CAD build for the part. Positions are in the model's coordinates, mm. A direction names the side the tool comes from. Round coordinates to 2 decimals unless told otherwise and drop trailing zeros. Order: outer loops, then holes, each group sorted by start corner. A loop starts at its lowest first (then second) coordinate and runs counter-clockwise, first axis right, second up. Notation, with made-up numbers: M 48,-30.75 L 93,-30.75 A21 cw 93,-3.75 Z; hole C -21,60 d1. An arc over 180 degrees is marked long. Put each result on its own line as item: value.
Autodesk Inventor part; units mm, degrees
ref_plane "YZ Plane" through (0, 0, 0) normal (1, 0, 0) x (0, 1, 0)
ref_plane "XZ Plane" through (0, 0, 0) normal (0, 1, 0) x (-1, 0, 0)
ref_plane "XY Plane" through (0, 0, 0) normal (0, 0, 1) x (1, 0, 0)
sketch "Sketch1" plane through (0, 0, 0) normal (0, 0, 1) x (1, 0, 0)
  circle A0 centre (-3.2581, -3.2482) radius 0.75
  circle A1 centre (11.7419, -13.2482) radius 0.75
  arc A2 (11.7419, -16.7482) -> (11.7419, -9.7482) centre (11.7419, -13.2482) ccw
  arc A3 (0.2419, -3.2482) -> (-6.7581, -3.2482) centre (-3.2581, -3.2482) ccw
  circle A4 centre (11.7419, -13.2482) radius 0.75
  circle A5 centre (-3.2581, -3.2482) radius 0.75
  line L0 (0.2419, -3.2482) -> (0.2419, -8.2482)
  line L1 (-6.7581, -3.2482) -> (-6.7581, -10.2482)
  line L2 (11.7419, -9.7482) -> (2.2419, -9.7482)
  line L3 (2.2419, -9.7482) -> (0.2419, -8.2482)
  line L4 (11.7419, -16.7482) -> (0.2419, -16.7482)
  line L5 (-6.7581, -10.2482) -> (0.2419, -16.7482)
  point P0 (0, 0)
  point P1 (-5.7424, -0.7828)
  point P2 (9.5175, -10.546)
  dimension "d0" = 7
  dimension "d1" = 7
  dimension "d4" = 5
  dimension "d5" = 7
  dimension "d6" = 9.5
  dimension "d7" = 11.5
  dimension "d8" = 15
extrude "Extrusion1" add sketch "Sketch1" against normal blind 4
properties part number "linkage"
Item 1: Mould opens along Y. For faces 1 (the cylindrical face through (-3.18, 0.25, -1.97)), 2 (the cylindrical face through (-2.85, -2.62, -1.97)), 3 (the flat face through (-3.31, -13.45, -1.97)), 4 (the cylindrical face through (12.15, -12.62, -1.97)) say: pulls with the +Y half, pulls with the -Y half, needs draft (parallel to the pull), parting line crosses it, or undercut.
Answers below:
face 1: pulls with the +Y half
face 2: undercut
face 3: pulls with the -Y half
face 4: undercut
Item 2: Band-saw the part on B-B on z = -1. Give the cut face in (x, y).
Answers below:
outline: M -6.76,-10.25 L 0.24,-16.75 L 11.74,-16.75 A3.5 ccw 11.74,-9.75 L 2.24,-9.75 L 0.24,-8.25 L 0.24,-3.25 A3.5 ccw -6.76,-3.25 Z; hole C -3.26,-3.25 d1.5; hole C 11.74,-13.25 d1.5
Item 3: Band-saw the part on C-C on y = -3.5. Give the cut face in (x, z).
Answers below:
outline: M -6.76,-4 L -3.96,-4 L -3.96,0 L -6.76,0 Z; M -2.55,-4 L 0.24,-4 L 0.24,0 L -2.55,0 Z
Item 4: Probe line 1 along Y through (x, z) = (5.5, -2.65); line 2 along X through (y, z) = (-5, -2.1); line 3 along X through (y, z) = (-12.75, -0.65). List the from-to ranges inside material, lowest first. Write a range as [from, to].
Answers below:
line 1: [-16.75, -9.75]
line 2: [-6.76, 0.24]
line 3: [-4.06, 11.18], [12.3, 15.21]
Item 5: Band-saw the part on D-D on x = 8.75. Give the cut face in (y, z).
Answers below:
outline: M -16.75,-4 L -9.75,-4 L -9.75,0 L -16.75,0 Z
Item 6: Pin check, flat tips, straight feed: P1, Ø1.2, axis at x = 8.5, z = -1.5, coming from the +Y side; P2, Ø2, axis at y = -5.5, z = -3.5, coming from the +X side; P3, Ø1, axis at y = -12, z = -3, coming from the +X side. Stop position of each tip, or through.
Answers below:
P1: y = -9.75
P2: x = 0.24
P3: x = 15.16
Item 7: Tool access for faces 5 (the flat face through (2, -10, 0)), 6 (the flat face through (7, -9.748, -2)): list every direction of +Z, -Z, +X, -X, +Y, -Y with a clear straight run to the whole face (end or side of a thin tool).
Answers below:
face 5: +Z, +X, -X, +Y, -Y
face 6: +Z, -Z, +X, +Y
Item 8: Band-saw the part on A-A on x = 11.5. Give the cut face in (y, z).
Answers below:
outline: M -16.75,-4 L -13.96,-4 L -13.96,0 L -16.75,0 Z; M -12.54,-4 L -9.75,-4 L -9.75,0 L -12.54,0 Z
